```python
from build123d import *

# Parameters (mm, degrees)
CONG_3_R                     = 2
CONG_4_R                     = 1
CONG_5_R                     = 1
CHANFREIN2_SIZE              = 1
CHANFREIN3_SIZE              = 1
R_P_TITION_CIRCULAIRE1_COUNT = 4
CONG_6_R                     = 0.4
R_P_TITION_CIRCULAIRE2_COUNT = 4


with BuildPart() as part:
    # Esquisse1 → R_volution1 (revolve)
    with BuildSketch(Plane.XY):
        Polygon((0, 0), (0, 4), (25, 4), (25, 12.5), (27.8, 12.5), (27.8, 21), (177.8, 21), (177.8, 11), (179.8, 11), (179.8, 4), (194.8, 4), (194.8, 0), align=None)
    revolve(axis=Axis((194.8, 0, 0), (-1, 0, 0)))

    # Cong_3
    cong_3_edges = [part.edges().sort_by_distance(p)[0] for p in [
        (177.8, -21, 0),
    ]]
    fillet(cong_3_edges, radius=CONG_3_R)

    # Cong_4
    cong_4_edges = [part.edges().sort_by_distance(p)[0] for p in [
        (25, -12.5, 0),
    ]]
    fillet(cong_4_edges, radius=CONG_4_R)

    # Cong_5
    cong_5_edges = [part.edges().sort_by_distance(p)[0] for p in [
        (179.8, -11, 0),
    ]]
    fillet(cong_5_edges, radius=CONG_5_R)

    # Chanfrein2
    chanfrein2_edges = [part.edges().sort_by_distance(p)[0] for p in [
        (0, -4, 0),
    ]]
    chamfer(chanfrein2_edges, length=CHANFREIN2_SIZE)

    # Chanfrein3
    chanfrein3_edges = [part.edges().sort_by_distance(p)[0] for p in [
        (194.8, -4, 0),
    ]]
    chamfer(chanfrein3_edges, length=CHANFREIN3_SIZE)

    # Esquisse6 → Trou taraud_ M3x0.51 (revolve, cut)
    with BuildSketch(Plane(origin=(27.8, -0.248189437, 16), x_dir=(0, 0, 1), z_dir=(0, 1, 0))):
        Polygon((0, 0), (0, 9.251075774), (1.25, 8.5), (1.25, 0), align=None)
    trou_taraud_m3x0_51 = revolve(axis=Axis((21.45, -0.248189437, 16), (1, 0, 0)), mode=Mode.SUBTRACT)

    # R_p_tition circulaire1: Trou taraud_ M3x0.51 ×4 about axis
    r_p_tition_circulaire1_axis = Axis((0, 0, 0), (1, 0, 0))
    for i in range(1, R_P_TITION_CIRCULAIRE1_COUNT):
        add(trou_taraud_m3x0_51.rotate(r_p_tition_circulaire1_axis, i * 360 / R_P_TITION_CIRCULAIRE1_COUNT), mode=Mode.SUBTRACT)

    # Cong_6
    cong_6_edges = [part.edges().sort_by_distance(p)[0] for p in [
        (27.8, -21, 0),
    ]]
    fillet(cong_6_edges, radius=CONG_6_R)

    # Esquisse24 → Trou taraud_ M4x0.72 (revolve, cut)
    with BuildSketch(Plane(origin=(27.8, -12.923800799, 12.52898132), x_dir=(0, 0, 1), z_dir=(0, 1, 0))):
        Polygon((0, 0), (0, 13.491420021), (1.65, 12.5), (1.65, 0), align=None)
    trou_taraud_m4x0_72 = revolve(axis=Axis((21.45, -12.923800799, 12.52898132), (1, 0, 0)), mode=Mode.SUBTRACT)

    # R_p_tition circulaire2: Trou taraud_ M4x0.72 ×4 about axis
    r_p_tition_circulaire2_axis = Axis((0, 0, 0), (1, 0, 0))
    for i in range(1, R_P_TITION_CIRCULAIRE2_COUNT):
        add(trou_taraud_m4x0_72.rotate(r_p_tition_circulaire2_axis, i * 360 / R_P_TITION_CIRCULAIRE2_COUNT), mode=Mode.SUBTRACT)


solid = part.part
```
Source: CAD feature listing. Evaluate the final solid. Frame: model axes, mm. A direction names the side the tool comes from. Coordinates: 2 decimals unless noted, no trailing zeros. Write each loop counter-clockwise with the first axis right and the second up, starting at its lowest first coordinate (ties: lowest second). Pieces come first, ordered by that corner, then holes. Notation, with made-up numbers: (40.5, 20.25) - (93.5, 20.25) arc R14 cw to (93.5, 30.25) - close; hole circle Ø5 at (62, 80.5). An arc over 180 degrees is marked (long way). Answer as a JSON object with one key per item and string values.
Q1. First-contact query: pin 1 Ø4.5 at (y, z) = (12.53, 12.92) entering from +X; pin 2 Ø6 at (x, z) = (36.5, -6) entering from -Y; pin 3 Ø6 at (x, z) = (150.5, 7.5) entering from -Y; pin 4 Ø18.5 at (y, z) = (4.5, -3.5) entering from -X. Flat tips, straight axial feed; report the tip coordinate or a pass-through.
Ans:
{"pin 1": "stops at x = 177.8", "pin 2": "stops at y = -20.78", "pin 3": "stops at y = -20.51", "pin 4": "stops at x = 0"}
Q2. Draft query along Y for faces 1 (the cylindrical face through (103.03, 20.03, -6.31)), 2 (the flat face through (179.8, 4.3, -0.1)), 3 (the conical face through (41.119, 12.467, 12.644)). Return one class per face: released by +Y, released by -Y, zero draft, split by the parting line, or undercut.
Ans:
{"face 1": "split by the parting line", "face 2": "zero draft", "face 3": "undercut"}
Q3. Section query B-B, the plane x = 163.5. Output: boundary loops of the cut face in (y, z).
Ans:
{"outline": "circle Ø42 at (0, 0)"}
Q4. Section query A-A, the plane x = 183.5. Output: boundary loops of the cut face in (y, z).
Ans:
{"outline": "circle Ø8 at (0, 0)"}
Q5. Material intervals for line 1 (Y direction, x = 182, z = -0.5); line 2 (X direction, y = 8, z = 5.5); line 3 (X direction, y = -4.5, z = -14.5), sorted ascending. Write a range as [from, to].
Ans:
{"line 1": "y = [-3.97, 3.97]", "line 2": "x = [25, 179.8]", "line 3": "x = [27.8, 177.8]"}
Q6. Set-up query: faces 4 (the flat face through (0, 0, 0)), 5 (the cylindrical face through (33.962, 11.313, -12.171)), 6 (the flat face through (177.8, 8, 8)). Return all of +Z, -Z, +X, -X, +Y, -Y with unobstructed straight access to the full face (end or side cutting, diameter ignored); none if empty.
Ans:
{"face 4": "+Z, -Z, -X, +Y, -Y", "face 5": "-X", "face 6": "+X"}
